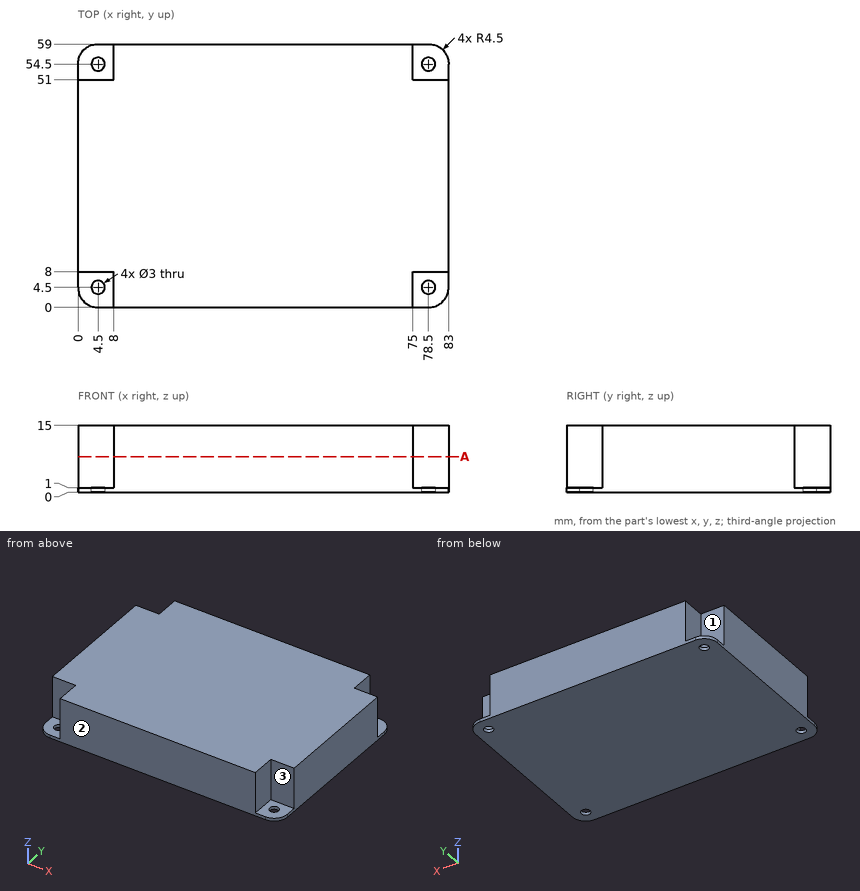
Study the drawing (mm; zero at the part's minimum x, y, z) and answer. A direction names the side the tool comes from. Round coordinates to 2 decimals unless told otherwise and drop trailing zeros. Write each loop counter-clockwise with the first axis right and the second up, starting at its lowest first coordinate (ties: lowest second). Pieces come first, ordered by that corner, then holes. Notation, with made-up numbers: (-24, 69.25) - (-2, 69.25) arc R16 cw to (-2, 81.25) - close; hole circle Ø1 at (-15.75, 27.25). An arc over 180 degrees is marked (long way). Use a Markdown table: item, result. Add a question column.
1. A tool of negligible diameter and unlimited length cuts with its end or side. For the marked faces 1, 2 and 3, from which of +Z, -Z, +X, -X, +Y, -Y can it reach the whole face along a straight path? Write none if from no direction.
2. The part is cut by section A-A (z = 8). Write down the section's boundary in (x, y).
3. Flat-ended cylindrical pins translate along their axes: P1, Ø6.5, axis at x = 80.5, z = 9.5, coming from the +Y side; P2, Ø6.5, axis at x = 2.5, z = 11.5, coming from the -Y side; P3, Ø2.5, axis at x = 4, y = 4.5, coming from the +Z side; P4, Ø1.8, axis at x = 4.5, y = 4.5, coming from the +Z side. Find the tip coordinate at first contact, or state that the pin passes through.
4. Consider line 1 (Y direction, x = 78.5, z = 0.5); line 2 (X direction, y = 6.5, z = 6.5); line 3 (Y direction, x = 77.5, z = 13.5). Determine where each line is inside the solid, lowest interval first.
Reported:
| question | item | result |
|---|---|---|
| 1 | face 1 | +Z, -X, +Y |
| 1 | face 2 | +Z, -Z, +X, -X, -Y |
| 1 | face 3 | +Z, +X, -Y |
| 2 | outline | (0, 8) - (8, 8) - (8, 0) - (75, 0) - (75, 8) - (83, 8) - (83, 51) - (75, 51) - (75, 59) - (8, 59) - (8, 51) - (0, 51) - close |
| 3 | P1 | y = 51 |
| 3 | P2 | y = 8 |
| 3 | P3 | z = 1 |
| 3 | P4 | through |
| 4 | line 1 | 0 to 3, 6 to 53, 56 to 59 |
| 4 | line 2 | 8 to 75 |
| 4 | line 3 | 8 to 51 |
